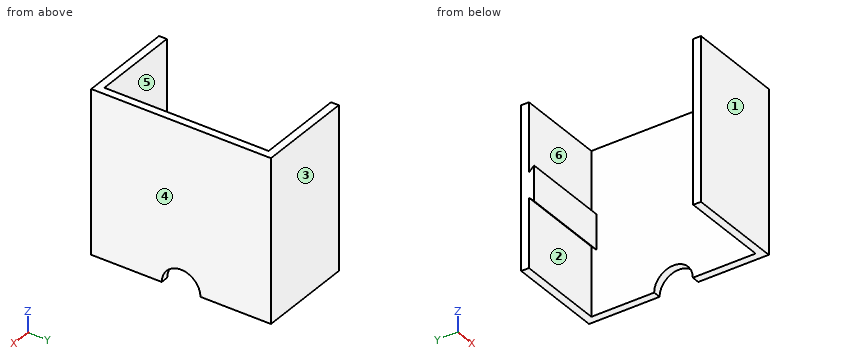
```python
from build123d import *

# Parameters (mm, degrees)
SKETCH1_W           = 42
SKETCH1_H           = 46.5
BOSS_EXTRUDE1_DEPTH = 2
SKETCH2_W           = 42
SKETCH2_H           = 2
BOSS_EXTRUDE2_DEPTH = 23
CUT_EXTRUDE1_DEPTH  = 23
BOSS_EXTRUDE3_DEPTH = 23


with BuildPart() as part:
    # Sketch1 → Boss-Extrude1 (new body)
    with BuildSketch(Plane(origin=(0, 0, 0), x_dir=(0, 0, -1), z_dir=(1, 0, 0))):
        Rectangle(SKETCH1_W, SKETCH1_H)
    extrude(amount=BOSS_EXTRUDE1_DEPTH)

    # Sketch2 → Boss-Extrude2 (add)
    with BuildSketch(Plane.ZY):
        with Locations((0, -22.25)):
            Rectangle(SKETCH2_W, SKETCH2_H)
    extrude(amount=BOSS_EXTRUDE2_DEPTH)

    # Sketch3 → Cut-Extrude1 (cut)
    with BuildSketch(Plane(origin=(2, 0, 0), x_dir=(0, 0, -1), z_dir=(1, 0, 0))):
        with BuildLine():
            Line((21, -5), (21, 5))
            ThreePointArc((21, 5), (16, 0), (21, -5))
        make_face()
    extrude(amount=-CUT_EXTRUDE1_DEPTH, mode=Mode.SUBTRACT)

    # Sketch4 → Boss-Extrude3 (add)
    with BuildSketch(Plane.ZY):
        Polygon((21, 23.25), (-21, 23.25), (-21, 21.25), (-3.2, 21.25), (-4.5, 19.95), (4.5, 19.95), (3.2, 21.25), (21, 21.25), align=None)
    extrude(amount=BOSS_EXTRUDE3_DEPTH)


solid = part.part
```
Can you work these out from the model? Positions are in its coordinate system, mm. Face numbers are marked on the shaded views. A direction names the side the tool comes from. Coordinates: 2 decimals unless noted, no trailing zeros. Loops run counter-clockwise (first coordinate to the right, second up) from the corner with the lowest first, then second, coordinate; pieces in that order, holes last.
1) For pin 1 (3 mm diameter, centred on y = 0.5, z = 11.5, fed in from -X), with a flat end and sliding along its axis, tell me the tip position at first contact or that it passes through.
2) Imagine slicing it at C-C on y = 0. List the corners of the cut face in (x, z) for me, plus the area to 3 significant figures.
3) Which directions (+Z, -Z, +X, -X, +Y, -Y) give clear straight access to the entire face, cutting with the end or side of a thin tool? Please do the marked faces 4, 5 and 6.
4) Imagine slicing it at B-B on z = 10.5. List the corners of the cut face in (x, y) for me, plus the area to 3 significant figures.
5) Imagine slicing it at D-D on z = -0.5. List the corners of the cut face in (x, y) for me.
6) I need wall thicknesses on probe 1 along Y at (x, z) = (-1.5, 2); probe 2 along Y at (x, z) = (-20.5, -14); probe 3 along X at (y, z) = (-14, 18). Which ranges of each line are inside material? Lowest first, please.
7) Imagine slicing it at A-A on x = -12.25. List the corners of the cut face in (y, z) for me, plus the area to 3 significant figures.
8) Thinking about a two-plate mould opening in Y: for the marked faces 1, 2 and 3, which applies, pulls with the +Y half, pulls with the -Y half, needs draft (parallel to the pull), parting line crosses it, or undercut?
Completed:
1. pin 1: stops at x = 0
2. outline: (0, -16) - (2, -16) - (2, 21) - (0, 21) - close
2. area: 74.0 mm2
3. face 4: +Z, -Z, +X, +Y, -Y
3. face 5: +Z, -Z, -X
3. face 6: +Z, -X
4. outline: (-23, -23.25) - (2, -23.25) - (2, 23.25) - (-23, 23.25) - (-23, 21.25) - (0, 21.25) - (0, -21.25) - (-23, -21.25) - close
4. area: 185 mm2
5. outline: (-23, -23.25) - (2, -23.25) - (2, 23.25) - (-23, 23.25) - (-23, 19.95) - (0, 19.95) - (0, -21.25) - (-23, -21.25) - close
6. probe 1: y = -23.25 to -21.25, 19.95 to 23.25
6. probe 2: y = -23.25 to -21.25, 21.25 to 23.25
6. probe 3: x = 0 to 2
7. outline: (-23.25, -21) - (-21.25, -21) - (-21.25, 21) - (-23.25, 21) - close; (19.95, -4.5) - (21.25, -3.2) - (21.25, -21) - (23.25, -21) - (23.25, 21) - (21.25, 21) - (21.25, 3.2) - (19.95, 4.5) - close
7. area: 178 mm2
8. face 1: pulls with the -Y half
8. face 2: undercut
8. face 3: pulls with the +Y half
